The listing builds one solid part. Answer for the finished solid, in the listing's coordinates (mm). A direction names the side the tool comes from. Coordinates: 2 decimals unless noted, no trailing zeros. Loops run counter-clockwise (first coordinate to the right, second up) from the corner with the lowest first, then second, coordinate; pieces in that order, holes last. Notation, with made-up numbers: M 48.5,63 L 62.5,63 A27 cw 62.5,88 Z; hole C -20,78 d11. An arc over 180 degrees is marked long. Answer in a Markdown table with one row per item. Add a question column.
from build123d import *

# Parameters (mm, degrees)
SALIENTE_EXTRUIR1_DEPTH      = 31.75
CORTAR_EXTRUIR1_REACH        = 93.76
CROQUIS5_R                   = 6.35
CORTAR_EXTRUIR2_REACH        = 65.52
CROQUIS6_R                   = 6.35
SALIENTE_EXTRUIR2_DEPTH      = 12.7
SALIENTE_EXTRUIR2_DEPTH_BACK = 38.1
CROQUIS7_R                   = 19.05
CROQUIS8_R                   = 9.525
CORTAR_EXTRUIR3_DEPTH        = 86.149806408


with BuildPart() as part:
    # Croquis3 → Saliente-Extruir1 (new body)
    with BuildSketch(Plane(origin=(0, 0, 0), x_dir=(0, 0, -1), z_dir=(1, 0, 0))):
        with BuildLine():
            Line((39.6875, 4.7625), (39.6875, -33.3375))
            Line((39.6875, -33.3375), (30.1625, -33.3375))
            Line((30.1625, -33.3375), (30.1625, -9.5885))
            ThreePointArc((30.1625, -9.5885), (28.748997326, -6.176002674), (25.3365, -4.7625))
            Line((25.3365, -4.7625), (-39.6875, -4.7625))
            Line((-39.6875, -4.7625), (-39.6875, 4.7625))
            Line((-39.6875, 4.7625), (39.6875, 4.7625))
        make_face()
    extrude(amount=SALIENTE_EXTRUIR1_DEPTH)

    # Croquis5 → Cortar-Extruir1 (cut, up to next)
    with BuildSketch(Plane(origin=(0, 0, -39.6875), x_dir=(-1, 0, 0), z_dir=(0, 0, -1)), mode=Mode.PRIVATE) as cortar_extruir1_sk1:
        with Locations((-15.875, -20.6375)):
            Circle(CROQUIS5_R)
    cortar_extruir1_tool1 = extrude(cortar_extruir1_sk1.sketch, amount=-CORTAR_EXTRUIR1_REACH, mode=Mode.PRIVATE) & part.part
    add(cortar_extruir1_tool1.solids().sort_by_distance((15.875, -20.6375, -39.6875))[0], mode=Mode.SUBTRACT)

    # Croquis6 → Cortar-Extruir2 (cut, up to next)
    with BuildSketch(Plane(origin=(0, 4.7625, 0), x_dir=(1, 0, 0), z_dir=(0, 1, 0)), mode=Mode.PRIVATE) as cortar_extruir2_sk1:
        with Locations(Location((15.875, 14.2875, 0), (0, 0, 270))):
            Circle(CROQUIS6_R)
    cortar_extruir2_tool1 = extrude(cortar_extruir2_sk1.sketch, amount=-CORTAR_EXTRUIR2_REACH, mode=Mode.PRIVATE) & part.part
    add(cortar_extruir2_tool1.solids().sort_by_distance((15.875, 4.7625, -14.2875))[0], mode=Mode.SUBTRACT)

    # Croquis7 → Saliente-Extruir2 (add, two sides: drawn at the far end of the back side and taken through both)
    with BuildSketch(Plane(origin=(0, 4.7625, 0), x_dir=(1, 0, 0), z_dir=(0, 1, 0)).offset(-SALIENTE_EXTRUIR2_DEPTH_BACK)):
        with Locations(Location((15.875, -39.6875, 0), (0, 0, 270))):
            Circle(CROQUIS7_R)
    extrude(amount=SALIENTE_EXTRUIR2_DEPTH + SALIENTE_EXTRUIR2_DEPTH_BACK)

    # Croquis8 → Cortar-Extruir3 (cut, through all)
    with BuildSketch(Plane(origin=(0, 17.4625, 0), x_dir=(1, 0, 0), z_dir=(0, 1, 0))):
        with Locations(Location((15.875, -39.6875, 0), (0, 0, 270))):
            Circle(CROQUIS8_R)
    extrude(amount=-CORTAR_EXTRUIR3_DEPTH, mode=Mode.SUBTRACT)


solid = part.part
(1) A cutting plane is placed at A-A (y = -25). State how many separate pieces and enclosed holes the cut face has, plus the area to 3 significant figures.
(2) Each of these flat-tipped pins is pushed along its axis until it touches: pin 1 (10 mm diameter, centred on y = 9.5, z = -20, fed in from +X); pin 2 (19 mm diameter, centred on y = -8, z = -15.5, fed in from -X); pin 3 (2 mm diameter, centred on x = 3.5, z = -27.5, fed in from -Y); pin 4 (11.5 mm diameter, centred on x = 15.88, z = 39.69, fed in from +Y). Where does it stop, or does it pass through?
(3) For faces 5 (the face through (0, -4, -13)), 6 (the face through (17.252, -26.836, -34.992)), 7 (the face through (25, 17.462, 44)), 8 (the face through (15.653, -6.214, -28.786)), determine the directions among +Z, -Z, +X, -X, +Y, -Y from which every point of the face is accessible in a straight line to the end or side of a thin tool.
(4) Straight lines are drawn through the part: line 1 (Z direction, x = 17, y = -3); line 2 (Z direction, x = 23, y = -28.5); line 3 (X direction, y = -26, z = -32). For each, find the intervals that lie inside material, in ascending order.
(5) The mould has two halves that part along Z. Classify faces 1 (the face through (12, -27, -30.162)), 2 (the face through (31.75, -4, -13)), 3 (the face through (16.29, -7.58, 30.17)), 4 (the face through (16, -14, -39.688)): released by +Z, released by -Z, zero draft, split by the parting line, or undercut.
(6) A cutting plane is placed at D-D (x = 13). Give the vertices of the cut face in (y, z).
(7) A cutting plane is placed at B-B (z = -19). Give the vertices of the cut face in (x, y), plus the area to 3 significant figures.
Solved:
| question | item | result |
|---|---|---|
| 1 | separate pieces | 3 |
| 1 | enclosed holes | 1 |
| 1 | area | 1,070 mm² |
| 2 | pin 1 | stops at x = 31.75 |
| 2 | pin 2 | stops at x = 0 |
| 2 | pin 3 | stops at y = -5.94 |
| 2 | pin 4 | passes through |
| 3 | face 5 | -Z, -X, +Y, -Y |
| 3 | face 6 | -Z |
| 3 | face 7 | +Z, -Z, +X, -X, +Y |
| 3 | face 8 | +X, -X, -Y |
| 4 | line 1 | z = -39.69 to -20.54, -8.04 to 30.23, 49.15 to 58.7 |
| 4 | line 2 | z = -39.69 to -30.16, 22.02 to 33.37, 46.01 to 57.35 |
| 4 | line 3 | x = 0 to 12.47, 19.28 to 31.75 |
| 5 | face 1 | undercut |
| 5 | face 2 | zero draft |
| 5 | face 3 | undercut |
| 5 | face 4 | released by -Z |
| 6 | outline | M -33.34,-39.69 L -26.3,-39.69 L -26.3,-30.16 L -33.34,-30.16 Z; M -33.34,20.86 L -4.76,20.86 L -4.76,-8.63 L 4.76,-8.63 L 4.76,20.86 L 17.46,20.86 L 17.46,30.61 L -33.34,30.61 Z; M -33.34,48.77 L 17.46,48.77 L 17.46,58.52 L -33.34,58.52 Z; M -14.98,-39.69 L 4.76,-39.69 L 4.76,-19.95 L -4.76,-19.95 L -4.76,-25.34 A4.83 cw -9.59,-30.16 L -14.98,-30.16 Z |
| 7 | outline | M 0,-4.76 L 11.62,-4.76 L 11.62,4.76 L 0,4.76 Z; M 20.13,-4.76 L 31.75,-4.76 L 31.75,4.76 L 20.13,4.76 Z |
| 7 | area | 221 mm² |
